```python
from build123d import *

# Parameters (mm, degrees)
SKETCH1_W                = 32
SKETCH1_H                = 70
BOSS_EXTRUDE1_DEPTH      = 40
BOSS_EXTRUDE1_DEPTH_BACK = 84.1
SKETCH2_W                = 21
SKETCH2_H                = 21
CUT_EXTRUDE1_DEPTH       = 17
CUT_EXTRUDE1_DEPTH_BACK  = 17
CUT_EXTRUDE2_START       = -18.5
SKETCH3_W                = 22
SKETCH3_H                = 45
CUT_EXTRUDE2_DEPTH       = 18.5
SKETCH4_W                = 42
SKETCH4_H                = 22
BOSS_EXTRUDE2_DEPTH      = 22
SKETCH5_R                = 2.75
CUT_EXTRUDE3_DEPTH       = 66.6
SKETCH6_W                = 7
SKETCH6_H                = 65
BOSS_EXTRUDE3_DEPTH      = 20
SKETCH7_R                = 2.5
CUT_EXTRUDE4_DEPTH       = 17
CUT_EXTRUDE4_DEPTH_BACK  = 39
SKETCH8_R                = 2.5
CUT_EXTRUDE5_DEPTH       = 8
FILLET1_R                = 2
FILLET2_R                = 5
SKETCH9_R                = 2.5
CUT_EXTRUDE6_DEPTH       = 47.45


with BuildPart() as part:
    # Sketch1 → Boss-Extrude1 (new body, two sides)
    with BuildSketch(Plane(origin=(0, 0, 0), x_dir=(1, 0, 0), z_dir=(0, 1, 0))) as boss_extrude1_sk:
        Rectangle(SKETCH1_W, SKETCH1_H)
    extrude(amount=BOSS_EXTRUDE1_DEPTH)
    extrude(boss_extrude1_sk.sketch, amount=-BOSS_EXTRUDE1_DEPTH_BACK)

    # Sketch2 → Cut-Extrude1 (cut, two sides)
    with BuildSketch(Plane(origin=(0, 0, 0), x_dir=(0, 0, -1), z_dir=(1, 0, 0))) as cut_extrude1_sk:
        with Locations((-24.5, 10.5)):
            Rectangle(SKETCH2_W, SKETCH2_H)
    extrude(amount=CUT_EXTRUDE1_DEPTH, mode=Mode.SUBTRACT)
    extrude(cut_extrude1_sk.sketch, amount=-CUT_EXTRUDE1_DEPTH_BACK, mode=Mode.SUBTRACT)

    # Sketch3 → Cut-Extrude2 (cut)
    with BuildSketch(Plane(origin=(0, 40, 0), x_dir=(1, 0, 0), z_dir=(0, 1, 0)).offset(CUT_EXTRUDE2_START)):
        with Locations((5, 12.5)):
            Rectangle(SKETCH3_W, SKETCH3_H)
    extrude(amount=CUT_EXTRUDE2_DEPTH, mode=Mode.SUBTRACT)

    # Sketch4 → Boss-Extrude2 (add)
    with BuildSketch(Plane(origin=(16, 0, 0), x_dir=(0, 0, -1), z_dir=(1, 0, 0))):
        with Locations((14, -29.5)):
            Rectangle(SKETCH4_W, SKETCH4_H)
    extrude(amount=BOSS_EXTRUDE2_DEPTH)

    # Sketch5 → Cut-Extrude3 (cut, through all)
    with BuildSketch(Plane(origin=(0, -18.5, 0), x_dir=(1, 0, 0), z_dir=(0, 1, 0))):
        with Locations((28.5, 18)):
            Circle(SKETCH5_R)
    extrude(amount=-CUT_EXTRUDE3_DEPTH, mode=Mode.SUBTRACT)

    # Sketch6 → Boss-Extrude3 (add)
    with BuildSketch(Plane.XY.offset(-35)):
        with Locations((-12.5, 7.5)):
            Rectangle(SKETCH6_W, SKETCH6_H)
    extrude(amount=-BOSS_EXTRUDE3_DEPTH)

    # Sketch7 → Cut-Extrude4 (cut, two sides)
    with BuildSketch(Plane.ZY) as cut_extrude4_sk:
        with Locations((24.5, -12)):
            Circle(SKETCH7_R)
    extrude(amount=CUT_EXTRUDE4_DEPTH, mode=Mode.SUBTRACT)
    extrude(cut_extrude4_sk.sketch, amount=-CUT_EXTRUDE4_DEPTH_BACK, mode=Mode.SUBTRACT)

    # Sketch8 → Cut-Extrude5 (cut, through all)
    with BuildSketch(Plane(origin=(-9, 0, 0), x_dir=(0, 0, -1), z_dir=(1, 0, 0))):
        with Locations((45, 25)):
            Circle(SKETCH8_R)
        with Locations((45, -10)):
            Circle(SKETCH8_R)
    extrude(amount=-CUT_EXTRUDE5_DEPTH, mode=Mode.SUBTRACT)

    # Fillet1
    fillet1_edges = [part.edges().sort_by_distance(p)[0] for p in [
        (-9, 7.5, -35),
    ]]
    fillet(fillet1_edges, radius=FILLET1_R)

    # Fillet2
    fillet2_edges = [part.edges().sort_by_distance(p)[0] for p in [
        (16, -18.5, -14),
        (16, -40.5, -14),
        (-12.5, -25, -35),
    ]]
    fillet(fillet2_edges, radius=FILLET2_R)

    # Sketch9 → Cut-Extrude6 (cut)
    with BuildSketch(Plane(origin=(0, 21.5, 0), x_dir=(1, 0, 0), z_dir=(0, 1, 0))):
        with Locations((6.5, 3.75)):
            Circle(SKETCH9_R)
    extrude(amount=-CUT_EXTRUDE6_DEPTH, mode=Mode.SUBTRACT)


solid = part.part
```
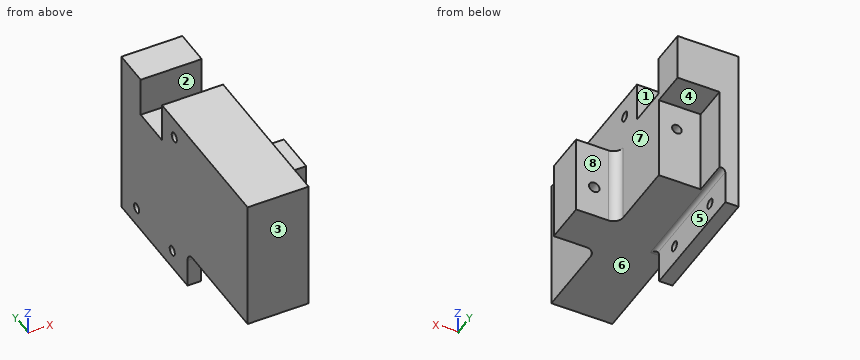
Could you check a few things on this model? Use its own coordinates, in mm. Face numbers are marked on the shaded views. A direction names the side the tool comes from. Round coordinates to 2 decimals unless told otherwise and drop trailing zeros. Loops run counter-clockwise (first coordinate to the right, second up) from the corner with the lowest first, then second, coordinate; pieces in that order, holes last. Notation, with made-up numbers: (66, 61) - (71, 61) arc R19 ccw to (71, 85) - close; hole circle Ø11 at (79, -33.75). An arc over 180 degrees is marked (long way). Answer in a Markdown table with one row per item. Add a question column.
(1) If we section it at B-B (z = 17): Please give me the cut outline in (x, y).
(2) If we section it at C-C (y = -37): Please give me the cut outline in (x, z), plus the area to 3 significant figures.
(3) If we section it at A-A (y = 25): Please give me the cut outline in (x, z), plus the area to 3 significant figures.
(4) If we mould it in two halves opening along Y, with no side actions, what happens to the marked faces 1, 2, 3 and 4? For each: pulls with the +Y half, pulls with the -Y half, needs draft (parallel to the pull), parting line crosses it, or undercut.
(5) If we section it at D-D (x = 28.5): Please give me the cut outline in (y, z).
(6) For the marked faces 5, 6, 7 and 8, which set-ups out of +Z, -Z, +X, -X, +Y, -Y let a thin tool reach every point of the face, with its end or its side?
(7) I'm going to push flat-ended pins straight in: pin 1 (8 mm diameter, centred on x = 21, z = -11, fed in from -Y); pin 2 (7.5 mm diameter, centred on x = -13.5, z = -50.5, fed in from -Y); pin 3 (1.5 mm diameter, centred on x = -6, y = -71, fed in from -Z); pin 4 (8 mm diameter, centred on x = 1.5, y = 19.5, fed in from +Z). Where does each tip first touch, or does it pass through?
(8) I need wall thicknesses on line 1 along Y through (x, z) = (-14, -45); line 2 along Y through (x, z) = (11, 31.5); line 3 along Z through (x, y) = (28.5, -31.5). Which ranges of each line are inside material? Lowest first, please.
Model answer:
| question | item | result |
|---|---|---|
| 1 | outline | (-16, -84.1) - (16, -84.1) - (16, 0) - (-16, 0) - close; (-16, 21) - (16, 21) - (16, 40) - (-16, 40) - close |
| 2 | outline | (-16, -35) - (38, -35) - (38, 7) - (16, 7) - (16, 35) - (-16, 35) - close; hole circle Ø5.5 at (28.5, -18) |
| 2 | area | 3,140 mm² |
| 3 | outline | (-16, -55) - (-9, -55) - (-9, -47.5) - (-16, -47.5) - close; (-16, -42.5) - (-9, -42.5) - (-9, -37) arc R2 cw to (-7, -35) - (-6, -35) - (-6, 10) - (16, 10) - (16, 35) - (-16, 35) - close |
| 3 | area | 1,360 mm² |
| 4 | face 1 | undercut |
| 4 | face 2 | undercut |
| 4 | face 3 | pulls with the -Y half |
| 4 | face 4 | needs draft |
| 5 | outline | (-40.5, -35) - (-18.5, -35) - (-18.5, -20.75) - (-40.5, -20.75) - close; (-40.5, -15.25) - (-18.5, -15.25) - (-18.5, 7) - (-40.5, 7) - close |
| 6 | face 5 | -Z, +X, +Y, -Y |
| 6 | face 6 | -Z, +X, -Y |
| 6 | face 7 | +Z, +X |
| 6 | face 8 | +Z, -Z, +X, +Y |
| 7 | pin 1 | stops at y = -42.5 |
| 7 | pin 2 | stops at y = -25 |
| 7 | pin 3 | stops at z = -35 |
| 7 | pin 4 | stops at z = 35 |
| 8 | line 1 | y = -25 to -12.5, -7.5 to 22.5, 27.5 to 40 |
| 8 | line 2 | y = -84.1 to 0, 21 to 40 |
| 8 | line 3 | z = -35 to -20.75, -15.25 to 7 |
